CAD build for the part. Positions are in the model's coordinates, mm. A direction names the side the tool comes from. Coordinates: 2 decimals unless noted, no trailing zeros. Write each loop counter-clockwise with the first axis right and the second up, starting at its lowest first coordinate (ties: lowest second). Pieces come first, ordered by that corner, then holes. Notation, with made-up numbers: (-9, -37) -> (16, -37) arc R19 ccw to (16, -18) -> close; hole circle Ø4 at (58.25, -33.5). An arc over 180 degrees is marked (long way). Answer as CSV lines item,"result".
Autodesk Fusion 360 part; units mm, degrees
sketch "Sketch1" plane through (0, 0, 0) normal (1, 0, 0) x (0, 1, 0)
  line L0 (0, 0) -> (25, 0)
  line L1 (25, 0) -> (25, 18)
  line L2 (0, 18) -> (0, 0)
  line L3 (19.25, 15) -> (19.25, 13)
  line L4 (19.25, 13) -> (5.75, 13)
  line L5 (5.75, 13) -> (5.75, 15)
  line L6 (18.25, 18) -> (18.25, 15)
  line L7 (6.75, 15) -> (6.75, 18)
  line L8 (25, 18) -> (18.25, 18)
  line L9 (6.75, 18) -> (0, 18)
  line L10 (5.75, 15) -> (6.75, 15)
  line L11 (18.25, 15) -> (19.25, 15)
  line L12 (6.75, 15) -> (18.25, 15)
  line L13 (5.75, 13) -> (19.25, 13)
  line L14 (19.25, 13) -> (19.25, 18)
  line L15 (19.25, 18) -> (5.75, 18)
  line L16 (5.75, 18) -> (5.75, 13)
  dimension "d1" = 25
  dimension "d2" = 18
  dimension "d3" = 13.5
  dimension "d4" = 2
  dimension "d5" = 13
  dimension "d6" = 5.75
  dimension "d7" = 1
  dimension "d8" = 11.5
  dimension "d9" = 3
  dimension "d10" = 15
  dimension "d32" = 13.5
sketch "Bokorys" plane through (0, 0, 0) normal (0, 1, 0) x (1, 0, 0)
  line L0 (-15, 0) -> (52, 0)
  line L1 (52, 0) -> (52, -6)
  line L2 (-15, -6) -> (-15, 0)
  line L3 (-15, -6) -> (52, -6)
  dimension "d48" = 15
  dimension "d49" = 67
  dimension "d50" = 6
extrude "Extrude1" add sketch "Sketch1" along normal blind 15 contours L0 L1 L2 L3 L4 L5 L8 L9 L13 L14 L16 | L7 L9 L10 L15 L16 | L6 L8 L11 L14 L15 makes body 1
extrude "Extrude2" add sketch "Sketch1" along normal blind 5 contours L3 L4 L5 L10 L11 L12 L13 L14 L16 bodies 1
extrude "Extrude3" add sketch "Sketch1" along normal blind 25 contours L0 L1 L2 L3 L4 L5 L8 L9 L13 L14 L16 bodies 1
extrude "Extrude4" add 1 faces at (25, 10.25, 4.3333) along direction (1, 0, 0) blind 2 on bodies 1 bodies 1
sketch "Sketch4" plane through (27, 0, 0) normal (1, 0, 0) x (0, 1, 0)
  line L0 (0, 18) -> (0, 0)
  line L1 (0, 0) -> (25, 0)
  line L2 (25, 0) -> (25, 18)
  line L3 (25, 18) -> (19.25, 18)
  line L4 (19.25, 18) -> (19.25, 13)
  line L5 (19.25, 13) -> (5.75, 13)
  line L6 (5.75, 13) -> (5.75, 18)
  line L7 (5.75, 18) -> (0, 18)
  line L8 (0, 0) -> (25, 0)
  line L9 (25, 0) -> (25, 18)
  line L10 (25, 18) -> (0, 18)
  line L11 (0, 18) -> (0, 0)
  circle A0 centre (12.5, 15.5) radius 1.25
  line L12 (10, 18) -> (15, 18)
  line L13 (15, 18) -> (15, 13)
  line L14 (15, 13) -> (10, 13)
  line L15 (10, 13) -> (10, 18)
  dimension "d39" = 2.5
  dimension "d40" = 2.5
  dimension "d41" = 25
  dimension "d42" = 12.5
  dimension "d57" = 13
  dimension "d59" = 2.5
  dimension "d60" = 5
  dimension "d61" = 5
extrude "Extrude5" add sketch "Sketch4" along normal blind 5 separate body contours L0 L1 L2 L3 L4 L5 L6 L7 L8 L9 L10 L11 L14 | L5 L6 L10 L15 | L5 L10 L12 L13 L14 L15 | L4 L5 L10 L13 | A0 makes body 2
extrude "Extrude6" add sketch "Sketch4" against normal blind 3 separate body contours A0 makes body 3
extrude "Extrude7" cut 1 faces at (24, 12.8855, 15.0845) along direction (1, 0, 0) blind 1 on bodies 3 bodies 3
extrude "Extrude8" add sketch "Bokorys" along normal blind 25 separate body makes body 4
combine "Combine1" operation add target body 4 tool bodies 2 1
fillet "Fillet1" radius 3 1 edges at (32, 12.5, 6) on bodies 4
fillet "Fillet2" radius 3 1 edges at (0, 12.5, 6) on bodies 4
extrude "Extrude9" add sketch "Sketch4" along normal blind 5 contours L5 L10 L12 L13 L14 L15 | A0 bodies 3
extrude "Extrude10" cut sketch "Sketch4" along normal blind 5 contours L5 L6 L10 L15 | L4 L5 L10 L13 bodies 4
fillet "Fillet3" radius 2 1 edges at (29.5, 10, 13) on bodies 4
fillet "Fillet4" radius 2 1 edges at (29.5, 15, 13) on bodies 4
combine "Combine2" operation add target body 4 tool bodies 3
move_face "OffsetFaces1" offset 5 1 faces at (32, 1.9167, 13.3333) on bodies 4
move_face "OffsetFaces2" offset -5 1 faces at (27, 12.4689, 17.5822) on bodies 4
move_face "OffsetFaces3" offset -5 1 faces at (25, 12.8855, 15.0845) on bodies 4
sketch "Sketch6" plane through (0, 0, 6) normal (0, 0, 1) x (-1, 0, 0)
  line L0 (3, 0) -> (3, -25)
  line L1 (3, -25) -> (15, -25)
  line L2 (15, -25) -> (15, 0)
  line L3 (15, 0) -> (3, 0)
  line L4 (15, -25) -> (-52, -25)
  line L5 (-52, -25) -> (-52, 0)
  line L6 (-52, 0) -> (15, 0)
  line L7 (15, 0) -> (15, -25)
  circle A0 centre (7.5, -12.5) radius 1.75
  line L8 (-18.5, -37) -> (-18.5, 8) construction
  circle A1 centre (-44.5, -12.5) radius 1.75
  dimension "d73" = 3.5
  dimension "d74" = 12.5
  dimension "d75" = 7.5
  dimension "d76" = 33.5
  dimension "d77" = 67
extrude "Extrude13" cut sketch "Sketch6" against normal blind 16 contours A0 | A1 bodies 4
extrude "Extrude11" [suppressed]
extrude "Extrude12" [suppressed]
Item 1: Saw through at B-B on x = -7.5. Give the cut face in (y, z).
Answer below:
outline,"(0, 0) -> (10.75, 0) -> (10.75, 6) -> (0, 6) -> close; (14.25, 0) -> (25, 0) -> (25, 6) -> (14.25, 6) -> close"
Item 2: Saw through at C-C on x = 6. Give the cut face in (y, z).
Answer below:
outline,"(0, 0) -> (25, 0) -> (25, 18) -> (18.25, 18) -> (18.25, 15) -> (19.25, 15) -> (19.25, 13) -> (5.75, 13) -> (5.75, 15) -> (6.75, 15) -> (6.75, 18) -> (0, 18) -> close"
Item 3: Wall check: line 1 (X direction, y = 12.5, z = 2.2); line 2 (Y direction, x = 44.5, z = 2.1); line 3 (Y direction, x = 31.5, z = 15). Give the ranges that are in metal, low to high. Write a range as from..to.
Answer below:
line 1,"x = -15..-9.25, -5.75..42.75, 46.25..52"
line 2,"y = 0..10.75, 14.25..25"
line 3,"y = 0..5.75, 11.35..13.65, 19.25..25"
Item 4: Flat gauge pins, fed straight in: pin 1 (1.5 mm diameter, centred on x = 23.5, y = 11, fed in from +Z); pin 2 (2 mm diameter, centred on y = 5, z = 8.5, fed in from -X); pin 3 (5.5 mm diameter, centred on y = 14, z = 16.5, fed in from -X). Where does each tip first touch, or does it go through?
Answer below:
pin 1,"stops at z = 13"
pin 2,"stops at x = -0.4"
pin 3,"stops at x = 0"
Item 5: 3-axis set-ups, long thin cutter, end or side, ignore diameter. For faces 5 (the flat face through (34, 15, 17)), 6 (the flat face through (30, 12, 16)), 7 (the flat face through (24, 5.75, 15)), 8 (the flat face through (44, 12, 11)): which of +Z, -Z, +X, -X, +Y, -Y reach the whole face in a straight line?
Answer below:
face 5,"+Z, +X, -X"
face 6,"+Z"
face 7,"+X"
face 8,"+Z, +X, +Y, -Y"
Item 6: Two-plate mould, pull along Z, no slides. Class faces 1 (the flat face through (-10, 12, 6)), 2 (the flat face through (7, 6.75, 16)), 3 (the cylindrical face through (31.014, 11.579, 16.345)), 4 (the flat face through (18, 12, 0)): pulls with the +Z half, pulls with the -Z half, needs draft (parallel to the pull), parting line crosses it, or undercut.
Answer below:
face 1,"pulls with the +Z half"
face 2,"needs draft"
face 3,"undercut"
face 4,"pulls with the -Z half"
Item 7: Saw through at A-A on y = 12.5. Give the cut face in (x, z).
Answer below:
outline,"(-15, 0) -> (-9.25, 0) -> (-9.25, 6) -> (-15, 6) -> close; (-5.75, 0) -> (42.75, 0) -> (42.75, 6) -> (46.25, 6) -> (46.25, 0) -> (52, 0) -> (52, 11) -> (37, 11) -> (37, 18) -> (32, 18) -> (32, 16.75) -> (30, 16.75) -> (30, 14.25) -> (32, 14.25) -> (32, 13) -> (5, 13) -> (5, 15) -> (0, 15) -> (0, 9) arc R3 cw to (-3, 6) -> (-5.75, 6) -> close"
Item 8: Saw through at D-D on y = 22.5. Give the cut face in (x, z), and give its area (3 significant figures).
Answer below:
outline,"(-15, 0) -> (52, 0) -> (52, 11) -> (37, 11) -> (37, 18) -> (0, 18) -> (0, 9) arc R3 cw to (-3, 6) -> (-15, 6) -> close"
area,"923 mm2"
